Work out the finished part from the listing and answer in its coordinate system (mm). Give positions to 0.01 mm unless a question says otherwise; leave off trailing zeros. Loops run counter-clockwise (first coordinate to the right, second up) from the corner with the lowest first, then second, coordinate; pieces in that order, holes last. Notation, with made-up numbers: (6.25, -21.5) - (44.25, -21.5) arc R17 ccw to (44.25, 6.5) - close; hole circle Ø9 at (-13.5, 80.5). An arc over 180 degrees is marked (long way). One line per item, written item: value.
from build123d import *

# Parameters (mm, degrees)
F0_R     = 18
F1_DEPTH = 12.5
F2_R     = 10
F3_DEPTH = 25


# Not quite as in the source:
# - a feature names something its author has since deleted; it is built from what else it names


with BuildPart() as f1:
    # F0 (on Front) → F1 (new body, symmetric)
    with BuildSketch(Plane.XZ):
        with BuildLine():
            Line((56.9371554598, -75), (595.9911190147, -75))
            Line((595.9911190147, -75), (595.9911190147, -33))
            Line((595.9911190147, -33), (519.5849960263, -33))
            Line((519.5849960263, -33), (450, -33))
            ThreePointArc((450, -33), (345.7777045638, -0.7457623443), (269.8662378191, 77.6128487294))
            Line((269.8662378191, 77.6128487294), (100, 375))
            Line((100, 375), (0, 375))
            Line((0, 375), (-100, 375))
            Line((-100, 375), (-269.8662378191, 77.6128487294))
            ThreePointArc((-269.8662378191, 77.6128487294), (-345.7777045638, -0.7457623443), (-450, -33))
            Line((-450, -33), (-484.7924980132, -33))
            Line((-484.7924980132, -33), (-519.5849960263, -33))
            Line((-519.5849960263, -33), (-595.9911190147, -33))
            Line((-595.9911190147, -33), (-595.9911190147, -75))
            Line((-595.9911190147, -75), (-56.9371554598, -75))
            Line((-56.9371554598, -75), (-39.1645557923, -47.3871512706))
            Line((-39.1645557923, -47.3871512706), (3.3388429378, -47.3871512706))
            Line((3.3388429378, -47.3871512706), (39.1645557923, -47.3871512706))
            Line((39.1645557923, -47.3871512706), (56.9371554598, -75))
        make_face()
        with Locations((-102.5, 63)):
            Circle(F0_R, mode=Mode.SUBTRACT)
        with Locations((102.5, 63)):
            Circle(F0_R, mode=Mode.SUBTRACT)
        with BuildLine():
            ThreePointArc((-74.4771999255, 121.0282629209), (-77.4732139948, 114.0830094681), (-84.4753157308, 111.2223771768))
            Line((-84.4753157308, 111.2223771768), (-197.1059338565, 111.2223771768))
            ThreePointArc((-197.1059338565, 111.2223771768), (-205.7661878943, 116.2223771768), (-205.7661878943, 126.2223771768))
            Line((-205.7661878943, 126.2223771768), (-125.0655397306, 266))
            ThreePointArc((-125.0655397306, 266), (-121.4052856928, 269.6602540378), (-116.4052856928, 271))
            Line((-116.4052856928, 271), (-81.7615214746, 271))
            ThreePointArc((-81.7615214746, 271), (-74.622153766, 268.0021017359), (-71.7634056693, 260.8058857441))
            Line((-71.7634056693, 260.8058857441), (-74.4771999255, 121.0282629209))
        make_face(mode=Mode.SUBTRACT)
        with Locations((-102.5, 301)):
            Circle(F0_R, mode=Mode.SUBTRACT)
        with BuildLine():
            ThreePointArc((84.4753157308, 111.2223771768), (77.4732139948, 114.0830094681), (74.4771999255, 121.0282629209))
            Line((74.4771999255, 121.0282629209), (71.7634056693, 260.8058857441))
            ThreePointArc((71.7634056693, 260.8058857441), (74.622153766, 268.0021017359), (81.7615214746, 271))
            Line((81.7615214746, 271), (116.4052856928, 271))
            ThreePointArc((116.4052856928, 271), (121.4052856928, 269.6602540378), (125.0655397306, 266))
            Line((125.0655397306, 266), (205.7661878943, 126.2223771768))
            ThreePointArc((205.7661878943, 126.2223771768), (205.7661878943, 116.2223771768), (197.1059338565, 111.2223771768))
            Line((197.1059338565, 111.2223771768), (84.4753157308, 111.2223771768))
        make_face(mode=Mode.SUBTRACT)
        with Locations((102.5, 301)):
            Circle(F0_R, mode=Mode.SUBTRACT)
        with BuildLine():
            ThreePointArc((100, 375), (413.732568712, 250.914148912), (595.9911190147, -33))
            Line((595.9911190147, -33), (621.814123166, -33))
            ThreePointArc((621.814123166, -33), (432.1619331745, 268.1134366241), (101.6213617791, 399.9473683177))
            ThreePointArc((101.6213617791, 399.9473683177), (0, 404.6514727579), (-101.6213617791, 399.9473683177))
            ThreePointArc((-101.6213617791, 399.9473683177), (-432.1619331745, 268.1134366241), (-621.814123166, -33))
            Line((-621.814123166, -33), (-595.9911190147, -33))
            ThreePointArc((-595.9911190147, -33), (-413.732568712, 250.914148912), (-100, 375))
            Line((-100, 375), (0, 375))
            Line((0, 375), (100, 375))
        make_face()
        with BuildLine():
            Line((-595.9911190147, -75), (-595.9911190147, -33))
            Line((-595.9911190147, -33), (-621.814123166, -33))
            ThreePointArc((-621.814123166, -33), (-626.6847460238, -53.9163527136), (-630.7708927375, -75))
            Line((-630.7708927375, -75), (-595.9911190147, -75))
        make_face()
        with BuildLine():
            Line((595.9911190147, -33), (595.9911190147, -75))
            Line((595.9911190147, -75), (630.7708927375, -75))
            ThreePointArc((630.7708927375, -75), (626.6847460238, -53.9163527136), (621.814123166, -33))
            Line((621.814123166, -33), (595.9911190147, -33))
        make_face()
    extrude(amount=F1_DEPTH, both=True)

    # F2
    f2_edges = [f1.edges().sort_by_distance(p)[0] for p in [
        (-100, 0, 375),
        (100, 0, 375),
        (595.991119, 0, -33),
        (-595.991119, 0, -33),
    ]]
    fillet(f2_edges, radius=F2_R)

    # F0 (on Front) → F3 (join, symmetric)
    with BuildSketch(Plane.XZ):
        Polygon((-484.7924980132, -33), (-450, -33), (-434.7924980132, -8), (-434.7924980132, 12), (-484.7924980132, 12), (-534.7924980132, 12), (-534.7924980132, -8), (-519.5849960263, -33), align=None)
        Polygon((37, -75), (56.9371554598, -75), (39.1645557923, -47.3871512706), (3.3388429378, -47.3871512706), (-39.1645557923, -47.3871512706), (-56.9371554598, -75), (-37, -75), (0, -75), align=None)
        Polygon((52, -103), (56.9371554598, -75), (37, -75), (37, -93), (27, -93), (27, -103), align=None)
        Polygon((-37, -93), (-37, -75), (-56.9371554598, -75), (-52, -103), (-27, -103), (-27, -93), align=None)
        Polygon((450, -33), (519.5849960263, -33), (534.7924980132, -8), (534.7924980132, 12), (484.7924980132, 12), (434.7924980132, 12), (434.7924980132, -8), align=None)
    extrude(amount=F3_DEPTH, both=True)


solid = f1.part
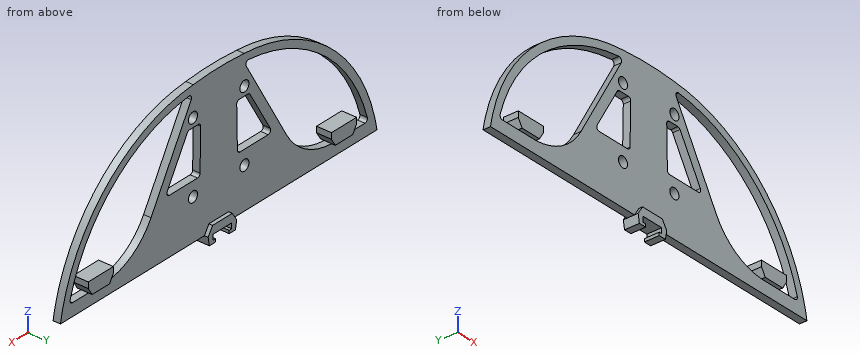
1. Section A-A (x = 492) is taken. Write down the section's boundary in (y, z), and give its area (3 significant figures).
Output:
outline: (-25, -33) - (-12.5, -33) - (-12.5, -75) - (12.5, -75) - (12.5, -33) - (25, -33) - (25, 12) - (-25, 12) - close; (-12.5, 171.99) - (12.5, 171.99) - (12.5, 210.51) - (-12.5, 210.51) - close
area: 4,260 mm²
2. Section D-D (y = -3) is taken. Count the separate pieces of the cut face and the enclosed holes in it, and give its area (3 significant figures).
Output:
separate pieces: 1
enclosed holes: 8
area: 251,000 mm²
3. Section B-B (z = 301) is taken. Write down the section's boundary in (x, y), and give its area (3 significant figures).
Output:
outline: (-388.6, -12.5) - (-341.86, -12.5) - (-341.86, 12.5) - (-388.6, 12.5) - close; (-142.27, -12.5) - (-120.5, -12.5) - (-120.5, 12.5) - (-142.27, 12.5) - close; (-84.5, -12.5) - (84.5, -12.5) - (84.5, 12.5) - (-84.5, 12.5) - close; (120.5, -12.5) - (142.27, -12.5) - (142.27, 12.5) - (120.5, 12.5) - close; (341.86, -12.5) - (388.6, -12.5) - (388.6, 12.5) - (341.86, 12.5) - close
area: 7,650 mm²
4. Section C-C (x = -138.5) is taken. Write down the section's boundary in (y, z).
Output:
outline: (-12.5, -75) - (12.5, -75) - (12.5, 111.22) - (-12.5, 111.22) - close; (-12.5, 242.73) - (12.5, 242.73) - (12.5, 307.6) - (-12.5, 307.6) - close; (-12.5, 371.13) - (12.5, 371.13) - (12.5, 396.35) - (-12.5, 396.35) - close
5. Find the intervals of material crossed by line 1 along Z through (x, y) = (-102.5, -3.25); line 2 along X through (y, z) = (7.5, 336); line 3 along X through (y, z) = (9.5, 231), in increasing order.
Output:
line 1: z = -75 to 45, 81 to 111.22, 271 to 283, 319 to 399.89
line 2: x = -330.2 to -270.63, -122.28 to 122.28, 270.63 to 330.2
line 3: x = -472.65 to -436.62, -182.25 to -145.27, -72.34 to 72.34, 145.27 to 182.25, 436.62 to 472.65
6. Flat-ended cylindrical pins translate along their axes: pin 1 Ø22 at (y, z) = (-7, -2.5) entering from +X; pin 2 Ø20 at (y, z) = (2, -88) entering from -X; pin 3 Ø11 at (y, z) = (1.5, -99) entering from -X; pin 4 Ø21.5 at (x, z) = (102.5, 63) entering from +Y. Find the tip coordinate at first contact, or state that the pin passes through.
Output:
pin 1: stops at x = 616.52
pin 2: stops at x = -56.41
pin 3: stops at x = -53.68
pin 4: passes through
